Input: part model. Units: mm. Frame: model coordinates. A direction names the side the tool comes from. Coordinates: 2 decimals unless noted, no trailing zeros. Order: outer loops, then holes, each group sorted by start corner. A loop starts at its lowest first (then second) coordinate and runs counter-clockwise, first axis right, second up.
from build123d import *

# Parameters (mm, degrees)
F0_R        = 4
F0_R_2      = 1.5
F1_DEPTH    = 10
F2_R        = 4
F3_DEPTH    = 2
F4_W        = 15
F4_H        = 1.5
F5_DEPTH    = 10
F6_T1_DEPTH = 4
F7_SIZE     = 5


# Not quite as in the source:
# - a fillet or chamfer that OpenCascade refuses, or shapes differently, is made with other operations: its cross-section is extruded or revolved along the edge and cut away or added


with BuildPart() as f1:
    # F0 (on Right) → F1 (new body)
    with BuildSketch(Plane.YZ):
        Circle(F0_R)
        Circle(F0_R_2, mode=Mode.SUBTRACT)
    extrude(amount=F1_DEPTH)

    # F2 (on face) → F3 (join)
    with BuildSketch(Plane.YZ.offset(10)):
        Circle(F2_R)
    extrude(amount=F3_DEPTH)

    # F4 (on Front) → F5 (join, symmetric)
    with BuildSketch(Plane.XZ):
        with Locations((15.5, 3.75)):
            Rectangle(F4_W, F4_H)
    extrude(amount=F5_DEPTH, both=True)

    # F6: fillet of radius 5 on 2 edges, made by hand

    # F6_s2 → F6_t1 (join)
    with BuildSketch(Plane.YZ.offset(8)):
        with BuildLine():
            ThreePointArc((-3.8999841722, -0.8888888889), (-5.6569165651, 1.9086797999), (-8.7749643874, 3))
            Line((-8.7749643874, 3), (-2.6457513111, 3))
            ThreePointArc((-2.6457513111, 3), (-3.8069052328, 1.2277917365), (-3.8999841722, -0.8888888889))
        make_face()
        with BuildLine():
            ThreePointArc((3.8999841722, -0.8888888889), (5.6569165651, 1.9086797999), (8.7749643874, 3))
            Line((8.7749643874, 3), (2.6457513111, 3))
            ThreePointArc((2.6457513111, 3), (3.8069052328, 1.2277917365), (3.8999841722, -0.8888888889))
        make_face()
    extrude(amount=F6_T1_DEPTH)

    # F7
    f7_edges = [f1.edges().sort_by_distance(p)[0] for p in [
        (8, 10, 3.75),
        (8, -10, 3.75),
    ]]
    chamfer(f7_edges, length=F7_SIZE)


solid = f1.part
Item 1: Cut plane C-C on y = 0. Return loops of the section in (x, z), then the cut area to 3 significant figures.
Response values:
outline: (0, -4) - (12, -4) - (12, 3) - (23, 3) - (23, 4.5) - (8, 4.5) - (8, 4) - (0, 4) - (0, 1.5) - (10, 1.5) - (10, -1.5) - (0, -1.5) - close
area: 84.5 mm2
Item 2: Pin query (flat end, axial travel): pin 1 Ø1.5 at (x, z) = (12.5, -2.5) entering from +Y; pin 2 Ø1.6 at (y, z) = (0, 1) entering from -X; pin 3 Ø1 at (x, z) = (9.5, 2.5) entering from +Y; pin 4 Ø5 at (x, y) = (13, 2.5) entering from -Z. Return the tip coordinate at first contact, or that it passes through.
Response values:
pin 1: stops at y = 3.5
pin 2: stops at x = 0
pin 3: stops at y = 6.97
pin 4: stops at z = -3.99
Item 3: Cut plane B-B on z = 2. Return loops of the section in (x, y), then the cut area to 3 significant figures.
Response values:
outline: (0, -3.46) - (8, -3.46) - (8, -5) - (8.77, -5.77) - (12, -5.77) - (12, 5.77) - (8.77, 5.77) - (8, 5) - (8, 3.46) - (0, 3.46) - close
area: 101 mm2
Item 4: Ray query, probe 1 along Z at (x, y) = (6, 0); probe 2 along X at (y, z) = (3, -2.5); probe 3 along X at (y, z) = (-4, 1.75). Return the intervals inside material, ascending.
Response values:
probe 1: z = -4 to -1.5, 1.5 to 4
probe 2: x = 0 to 12
probe 3: x = 8 to 12
Item 5: Cut plane A-A on x = 2. Return loops of the section in (y, z).
Response values:
outline: circle Ø8 at (0, 0); hole circle Ø3 at (0, 0)
Item 6: Draft query along Z for faces 1 (the face through (10.42, -5.08, 1.37)), 2 (the face through (10, -7, 4)), 3 (the face through (4.93, -1.5, 0.07)). Return one class per face: pulls with the +Z half, pulls with the -Z half, needs draft (parallel to the pull), parting line crosses it, or undercut.
Response values:
face 1: pulls with the -Z half
face 2: needs draft
face 3: undercut
Item 7: Access query for faces 4 (the face through (4.583, 1.846, -3.549)), 5 (the face through (0, 2, 0)), 6 (the face through (12, 0, 0)). Directions: +Z, -Z, +X, -X, +Y, -Y. A direction counts if a zero-diameter tool reaches every point of the face in a straight line with its end or side. Return the directions, or none.
Response values:
face 4: -X
face 5: +Z, -Z, -X, +Y, -Y
face 6: -Z, +X, +Y, -Y
Item 8: Cut plane D-D on x = 15.25. Return loops of the section in (y, z).
Response values:
outline: (-10, 3) - (10, 3) - (10, 4.5) - (-10, 4.5) - close
